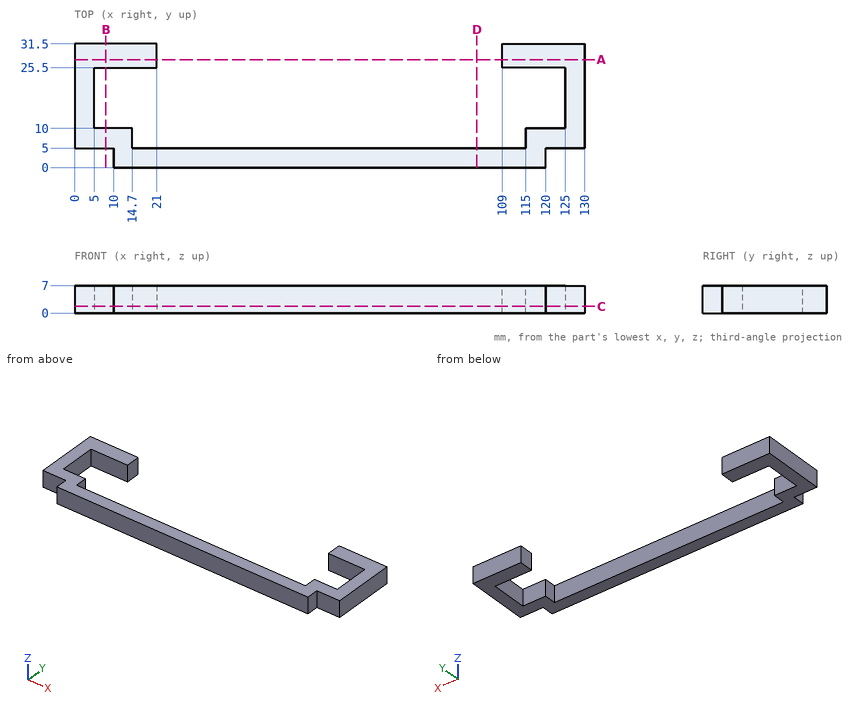
For this review, use the dimensioned drawing (mm, ordinates from the lowest corner) and the shaded views. Round coordinates to 2 decimals unless told otherwise and drop trailing zeros. Order: outer loops, then holes, each group sorted by start corner. A loop starts at its lowest first (then second) coordinate and runs counter-clockwise, first axis right, second up.
1) Consider section C-C (z = 1.75). State the section outline as (x, y) points, plus the area to 3 significant figures.
The answers:
outline: (0, 5) - (10, 5) - (10, 0) - (120, 0) - (120, 5) - (130, 5) - (130, 31.5) - (109, 31.5) - (109, 25.5) - (125, 25.5) - (125, 10) - (115, 10) - (115, 5) - (14.7, 5) - (14.7, 10) - (5, 10) - (5, 25.5) - (21, 25.5) - (21, 31.5) - (0, 31.5) - close
area: 1,110 mm2
2) For L1, parallel to X at y = 17.5, z = 3.25; L2, parallel to Y at x = 12, z = 1; L3, parallel to X at y = 26, z = 4, list the stretches that pass through material, from the lowest coordinate up.
The answers:
L1: x = 0 to 5, 125 to 130
L2: y = 0 to 10, 25.5 to 31.5
L3: x = 0 to 21, 109 to 130
3) Clearance check with flat-ended pins moving along their axes: pin 1 Ø8 at (x, y) = (57.5, 5) entering from -Z; pin 2 Ø2.5 at (y, z) = (2.5, 3) entering from -X. State where each tip first meets the part, or that it passes through.
The answers:
pin 1: stops at z = 0
pin 2: stops at x = 10
4) Consider section A-A (y = 27.5). State the section outline as (x, z) points.
The answers:
outline: (0, 0) - (21, 0) - (21, 7) - (0, 7) - close; (109, 0) - (130, 0) - (130, 7) - (109, 7) - close
5) Consider section D-D (x = 102.5). State the section outline as (y, z) points, plus the area to 3 significant figures.
The answers:
outline: (0, 0) - (5, 0) - (5, 7) - (0, 7) - close
area: 35.0 mm2
6) Consider section B-B (x = 8). State the section outline as (y, z) points.
The answers:
outline: (5, 0) - (10, 0) - (10, 7) - (5, 7) - close; (25.5, 0) - (31.5, 0) - (31.5, 7) - (25.5, 7) - close
